from build123d import *

# Parameters (mm, degrees)
CUT_EXTRUDE1_DEPTH      = 124.426091245
CUT_EXTRUDE1_DEPTH_BACK = 124.426091245
SKETCH2_R               = 8


with BuildPart() as part:
    # Sketch1 → Revolve1 (revolve)
    with BuildSketch(Plane.XY, mode=Mode.PRIVATE) as revolve1_sk:
        with BuildLine():
            Line((0, 45), (18, 45))
            Line((18, 45), (18, 85))
            Line((18, 85), (26, 85))
            ThreePointArc((26, 85), (27.414213562, 84.414213562), (28, 83))
            Line((28, 83), (28, 49.5))
            ThreePointArc((28, 49.5), (28.585786438, 48.085786438), (30, 47.5))
            Line((30, 47.5), (38.3, 47.5))
            ThreePointArc((38.3, 47.5), (39.714213562, 46.914213562), (40.3, 45.5))
            Line((40.3, 45.5), (40.3, 42.5))
            Line((40.3, 42.5), (30.3, 42.5))
            Line((30.3, 42.5), (30.3, 25.05))
            Line((30.3, 25.05), (20.3, 25.05))
            Line((20.3, 25.05), (20.3, 31))
            Line((20.3, 31), (14.35, 31))
            Line((14.35, 31), (13, 31.238041424))
            Line((13, 31.238041424), (13, 37))
            ThreePointArc((13, 37), (12.414213562, 38.414213562), (11, 39))
            Line((11, 39), (0, 39))
            Line((0, 39), (0, 45))
        make_face()
    revolve(revolve1_sk.sketch.rotate(Axis((0, 0, 0), (1, 0, 0)), 90), axis=Axis((0, 0, 0), (1, 0, 0)))

    # Sketch2 → Cut-Extrude1 (cut, two sides: drawn at the far end of the back side and taken through both)
    with BuildSketch(Plane(origin=(28, 0, 0), x_dir=(0, 0, -1), z_dir=(1, 0, 0)).offset(-CUT_EXTRUDE1_DEPTH_BACK)):
        with Locations((70, 0)):
            Circle(SKETCH2_R)
        with Locations((35, -60.621778265)):
            Circle(SKETCH2_R)
        with Locations((-35, -60.621778265)):
            Circle(SKETCH2_R)
        with Locations((-70, 0)):
            Circle(SKETCH2_R)
        with Locations((-35, 60.621778265)):
            Circle(SKETCH2_R)
        with Locations((35, 60.621778265)):
            Circle(SKETCH2_R)
    extrude(amount=CUT_EXTRUDE1_DEPTH + CUT_EXTRUDE1_DEPTH_BACK, mode=Mode.SUBTRACT)


solid = part.part
Model file for the job. Use its own axes, mm. A direction names the side the tool comes from. Round coordinates to 2 decimals unless told otherwise and drop trailing zeros. Order: outer loops, then holes, each group sorted by start corner. A loop starts at its lowest first (then second) coordinate and runs counter-clockwise, first axis right, second up.
(1) Band-saw the part on B-B (y = 0). Give the number of separate pieces and of enclosed holes in the cut face, then the cut area to 3 significant figures.
(2) 3-axis set-ups, long thin cutter, end or side, ignore diameter. For faces 4 (the face through (22.056, -25.532, 81.075)), 5 (the face through (5.423, -38.668, -5.077)), 6 (the face through (30.3, 18, 18)): which of +Z, -Z, +X, -X, +Y, -Y reach the whole face in a straight line?
(3) Band-saw the part on A-A (x = 23.5). List the corners of the cut face in (y, z).
(4) Drill centre lines: line 1 (Y direction, x = 26.25, z = 0); line 2 (Z direction, x = 20, y = -64); line 3 (Z direction, x = 19.5, y = -3). Where is each one in solid material? Low to high.
(5) Pull direction Z, two halves, no side cores. Call faces 1 (the face through (34.21, 46.37, -10.3)), 2 (the face through (13, 19, 25)), 3 (the face through (28, 36, 36)): released by +Z, released by -Z, zero draft, split by the parting line, or undercut.
(6) Pin check, flat tips, straight feed: pin 1 (8 mm diameter, centred on x = 12.5, y = 0, fed in from -Z); pin 2 (1.5 mm diameter, centred on y = 5.5, z = -41, fed in from -X); pin 3 (2 mm diameter, centred on y = 50, z = 9.5, fed in from +X); pin 4 (13 mm diameter, centred on y = -60.62, z = -35, fed in from -X). Stop position of each tip, or through.
(7) Band-saw the part on C-C (x = 4). List the corners of the cut face in (y, z).
Verdict:
1. separate pieces: 4
1. enclosed holes: 0
1. area: 1,350 mm2
2. face 4: +X, -X
2. face 5: -X
2. face 6: +X
3. outline: circle Ø170 at (0, 0); hole circle Ø16 at (-60.62, -35); hole circle Ø16 at (-60.62, 35); hole circle Ø50.1 at (0, 0); hole circle Ø16 at (0, -70); hole circle Ø16 at (0, 70); hole circle Ø16 at (60.62, -35); hole circle Ø16 at (60.62, 35)
4. line 1: y = -84.98 to -25.05, 25.05 to 84.98
4. line 2: z = -55.94 to -42.25, -27.75 to 27.75, 42.25 to 55.94
4. line 3: z = -84.95 to -77.42, -62.58 to -30.85, 30.85 to 62.58, 77.42 to 84.95
5. face 1: split by the parting line
5. face 2: undercut
5. face 3: zero draft
6. pin 1: stops at z = -45
6. pin 2: stops at x = 0
6. pin 3: stops at x = 28
6. pin 4: passes through
7. outline: circle Ø90 at (0, 0); hole circle Ø78 at (0, 0)
